from build123d import *

# Parameters (mm, degrees)
SKETCH_1_W      = 650
SKETCH_1_H      = 50
SKETCH_1_R      = 16.5
EXTRUDE_1_DEPTH = 50
FILLET_1_R      = 25


with BuildPart() as part:
    # 草图1 → 凸台-拉伸1 (new body)
    with BuildSketch(Plane(origin=(0, 0, 0), x_dir=(1, 0, 0), z_dir=(0, 1, 0))):
        with Locations((325, 25)):
            Rectangle(SKETCH_1_W, SKETCH_1_H)
        with Locations(Location((625, 25, 0), (0, 0, 270))):
            Circle(SKETCH_1_R, mode=Mode.SUBTRACT)
        with Locations(Location((325, 25, 0), (0, 0, 270))):
            Circle(SKETCH_1_R, mode=Mode.SUBTRACT)
    extrude(amount=EXTRUDE_1_DEPTH)

    # 圆角1
    fillet_1_edges = [part.edges().sort_by_distance(p)[0] for p in [
        (0, 25, -50),
        (0, 25, 0),
        (650, 25, -50),
        (650, 25, 0),
    ]]
    fillet(fillet_1_edges, radius=FILLET_1_R - 0.0001)  # a hair under: the kernel refuses the full size


solid = part.part
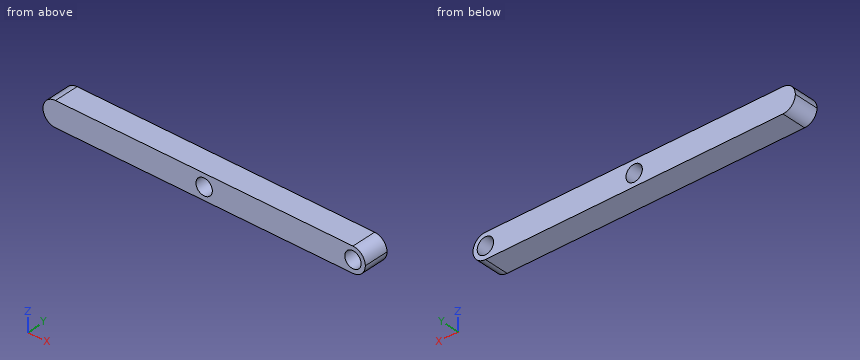
The listing builds one solid part. Answer for the finished solid, in the listing's coordinates (mm). Coordinates: 2 decimals unless noted, no trailing zeros. Write each loop counter-clockwise with the first axis right and the second up, starting at its lowest first coordinate (ties: lowest second). Pieces come first, ordered by that corner, then holes. Notation, with made-up numbers: M 64,-40 L 109,-40 A17 ccw 109,-17 Z; hole C 57.5,77.5 d11. An arc over 180 degrees is marked long. Write each question's results on one line, items separated by ' | '.
Item 1: The part is cut by section A-A on x = 325. Determine the outline of the cut face in (y, z).
Answer below:
outline: M 0,-50 L 50,-50 L 50,-41.5 L 0,-41.5 Z; M 0,-8.5 L 50,-8.5 L 50,0 L 0,0 Z
Item 2: The part is cut by section C-C on y = 10. State how many separate pieces and enclosed holes the cut face has, and give its area (3 significant figures).
Answer below:
separate pieces: 1 | enclosed holes: 2 | area: 30,300 mm2
Item 3: Given P1, Ø5, axis at y = 8.5, z = -20.5, coming from the -X side; P2, Ø6, axis at y = 39.5, z = -39.5, coming from the -X side; P3, Ø5, axis at x = 252, z = -39, coming from the -Y side; P4, Ø5, axis at y = 5.5, z = -32, coming from the +X side, each flat-ended and moving along its own axis, determine where each tip first touches the part or whether it passes through.
Answer below:
P1: x = 0.08 | P2: x = 2.8 | P3: y = 0 | P4: x = 649.59
Item 4: The part is cut by section B-B on z = -33. Determine the outline of the cut face in (x, y).
Answer below:
outline: M 1.31,0 L 310.57,0 L 310.57,50 L 1.31,50 Z; M 339.43,0 L 610.57,0 L 610.57,50 L 339.43,50 Z; M 639.43,0 L 648.69,0 L 648.69,50 L 639.43,50 Z
Item 5: Consider probe 1 along X at (y, z) = (24, -25); probe 2 along X at (y, z) = (19, -35); probe 3 along Z at (x, y) = (317, 29.5). Determine where each line is inside the solid, lowest interval first. Write a range as [from, to].
Answer below:
probe 1: [0, 308.5], [341.5, 608.5], [641.5, 650] | probe 2: [2.09, 311.88], [338.12, 611.88], [638.12, 647.91] | probe 3: [-50, -39.43], [-10.57, 0]
